from build123d import *

# Parameters (mm, degrees)
F0_W     = 50
F0_H     = 20
F1_DEPTH = 3


with BuildPart() as f1:
    # F0 (on Top) → F1 (new body)
    with BuildSketch(Plane.XY):
        Rectangle(F0_W, F0_H)
        Polygon((-13.6844948676, 3.9411129119), (-13.6844948676, -6.2236628849), (-16.3019989195, -6.2236628849), (-16.3019989195, 3.9411129119), (-19.6542409508, 3.9411129119), (-19.6542409508, 6.1183144246), (-10.3349540789, 6.1183144246), (-10.3349540789, 3.9411129119), align=None, mode=Mode.SUBTRACT)
        Polygon((-1.3290113452, -4.0626688277), (-1.3290113452, -6.2236628849), (-8.4359805511, -6.2236628849), (-8.4359805511, 6.1183144246), (-1.3290113452, 6.1183144246), (-1.3290113452, 3.9735278228), (-5.8184764992, 3.9735278228), (-5.8184764992, 1.2641815235), (-1.639654241, 1.2641815235), (-1.639654241, -0.8806050783), (-5.8184764992, -0.8806050783), (-5.8184764992, -4.0626688277), align=None, mode=Mode.SUBTRACT)
        with BuildLine():
            add(Edge.make_bspline(
                [(7.8889789303, -0.7576985413), (8.5305240411, -1.5883306321), (8.5305240411, -2.7957860616)],
                knots=[0, 0, 0, 1, 1, 1], degree=2))
            add(Edge.make_bspline(
                [(8.5305240411, -2.7957860616), (8.5305240411, -4.4678552134), (7.3271204754, -5.4308481902)],
                knots=[0, 0, 0, 1, 1, 1], degree=2))
            add(Edge.make_bspline(
                [(7.3271204754, -5.4308481902), (6.1237169098, -6.3938411669), (3.9816315505, -6.3938411669)],
                knots=[0, 0, 0, 1, 1, 1], degree=2))
            add(Edge.make_bspline(
                [(3.9816315505, -6.3938411669), (2.0043219881, -6.3938411669), (0.4862236629, -5.6482982172)],
                knots=[0, 0, 0, 1, 1, 1], degree=2))
            Line((0.4862236629, -5.6482982172), (0.4862236629, -3.2171799028))
            add(Edge.make_bspline(
                [(0.4862236629, -3.2171799028), (1.734197731, -3.7763371151), (2.5999459751, -4.0032414911)],
                knots=[0, 0, 0, 1, 1, 1], degree=2))
            add(Edge.make_bspline(
                [(2.5999459751, -4.0032414911), (3.4656942193, -4.2301458671), (4.1842247434, -4.2301458671)],
                knots=[0, 0, 0, 1, 1, 1], degree=2))
            add(Edge.make_bspline(
                [(4.1842247434, -4.2301458671), (5.0432198811, -4.2301458671), (5.5037817396, -3.9019448947)],
                knots=[0, 0, 0, 1, 1, 1], degree=2))
            add(Edge.make_bspline(
                [(5.5037817396, -3.9019448947), (5.9643435981, -3.5737439222), (5.9643435981, -2.9227444625)],
                knots=[0, 0, 0, 1, 1, 1], degree=2))
            add(Edge.make_bspline(
                [(5.9643435981, -2.9227444625), (5.9643435981, -2.5607779579), (5.7617504052, -2.2771474878)],
                knots=[0, 0, 0, 1, 1, 1], degree=2))
            add(Edge.make_bspline(
                [(5.7617504052, -2.2771474878), (5.5591572123, -1.9935170178), (5.1661264182, -1.7328471097)],
                knots=[0, 0, 0, 1, 1, 1], degree=2))
            add(Edge.make_bspline(
                [(5.1661264182, -1.7328471097), (4.773095624, -1.4721772015), (3.5656401945, -0.8968125338)],
                knots=[0, 0, 0, 1, 1, 1], degree=2))
            add(Edge.make_bspline(
                [(3.5656401945, -0.8968125338), (2.4365207996, -0.3646677472), (1.8706104808, 0.1242571583)],
                knots=[0, 0, 0, 1, 1, 1], degree=2))
            add(Edge.make_bspline(
                [(1.8706104808, 0.1242571583), (1.3047001621, 0.6131820637), (0.9670448406, 1.2641815235)],
                knots=[0, 0, 0, 1, 1, 1], degree=2))
            add(Edge.make_bspline(
                [(0.9670448406, 1.2641815235), (0.6293895192, 1.9151809833), (0.6293895192, 2.7822798487)],
                knots=[0, 0, 0, 1, 1, 1], degree=2))
            add(Edge.make_bspline(
                [(0.6293895192, 2.7822798487), (0.6293895192, 4.4219340897), (1.7396002161, 5.3579146407)],
                knots=[0, 0, 0, 1, 1, 1], degree=2))
            add(Edge.make_bspline(
                [(1.7396002161, 5.3579146407), (2.849810913, 6.2938951918), (4.8082117774, 6.2938951918)],
                knots=[0, 0, 0, 1, 1, 1], degree=2))
            add(Edge.make_bspline(
                [(4.8082117774, 6.2938951918), (5.7698541329, 6.2938951918), (6.6437061048, 6.0669908158)],
                knots=[0, 0, 0, 1, 1, 1], degree=2))
            add(Edge.make_bspline(
                [(6.6437061048, 6.0669908158), (7.5175580767, 5.8400864398), (8.4710967045, 5.4267963263)],
                knots=[0, 0, 0, 1, 1, 1], degree=2))
            Line((8.4710967045, 5.4267963263), (7.6283090222, 3.3900594273))
            add(Edge.make_bspline(
                [(7.6283090222, 3.3900594273), (6.639654241, 3.7952458131), (5.9940572663, 3.9559697461)],
                knots=[0, 0, 0, 1, 1, 1], degree=2))
            add(Edge.make_bspline(
                [(5.9940572663, 3.9559697461), (5.3484602917, 4.1166936791), (4.7244732577, 4.1166936791)],
                knots=[0, 0, 0, 1, 1, 1], degree=2))
            add(Edge.make_bspline(
                [(4.7244732577, 4.1166936791), (3.9816315505, 4.1166936791), (3.5845488925, 3.7709346299)],
                knots=[0, 0, 0, 1, 1, 1], degree=2))
            add(Edge.make_bspline(
                [(3.5845488925, 3.7709346299), (3.1874662345, 3.4251755808), (3.1874662345, 2.868719611)],
                knots=[0, 0, 0, 1, 1, 1], degree=2))
            add(Edge.make_bspline(
                [(3.1874662345, 2.868719611), (3.1874662345, 2.5229605619), (3.3481901675, 2.2649918963)],
                knots=[0, 0, 0, 1, 1, 1], degree=2))
            add(Edge.make_bspline(
                [(3.3481901675, 2.2649918963), (3.5089141005, 2.0070232307), (3.8587250135, 1.7666126418)],
                knots=[0, 0, 0, 1, 1, 1], degree=2))
            add(Edge.make_bspline(
                [(3.8587250135, 1.7666126418), (4.2085359265, 1.5262020529), (5.5159373312, 0.9022150189)],
                knots=[0, 0, 0, 1, 1, 1], degree=2))
            add(Edge.make_bspline(
                [(5.5159373312, 0.9022150189), (7.2474338196, 0.0729335494), (7.8889789303, -0.7576985413)],
                knots=[0, 0, 0, 1, 1, 1], degree=2))
        make_face(mode=Mode.SUBTRACT)
        Polygon((15.529443544, 3.9411129119), (15.529443544, -6.2236628849), (12.9119394922, -6.2236628849), (12.9119394922, 3.9411129119), (9.5596974608, 3.9411129119), (9.5596974608, 6.1183144246), (18.8789843328, 6.1183144246), (18.8789843328, 3.9411129119), align=None, mode=Mode.SUBTRACT)
    extrude(amount=F1_DEPTH)


solid = f1.part
The listing builds one solid part. Answer for the finished solid, in the listing's coordinates (mm). Round coordinates to 2 decimals unless told otherwise and drop trailing zeros. Order: outer loops, then holes, each group sorted by start corner. A loop starts at its lowest first (then second) coordinate and runs counter-clockwise, first axis right, second up. Notation, with made-up numbers: (81, -8) -> (102, -8) arc R33 ccw to (102, 23) -> close; hole circle Ø10 at (30, 61). An arc over 180 degrees is marked (long way). Put each result on its own line as item: value.
Q1. Consider line 1 along Y through (x, z) = (-11, 1.45); line 2 along Y through (x, z) = (1, 2); line 3 along X through (y, z) = (-2.5, 0.8). Determine where each line is inside the solid, lowest interval first.
Results list:
line 1: -10 to 3.94, 6.12 to 10
line 2: -10 to -5.87, -3.44 to 1.2, 4.44 to 10
line 3: -25 to -16.3, -13.68 to -8.44, -5.82 to 5.88, 8.52 to 12.91, 15.53 to 25
Q2. Determine the mould class of faces 1 (the flat face through (25, 0, 1)), 2 (the flat face through (0, -10, 1)), 3 (the flat face through (-1.64, 0, 1)) for opening direction Y: pulls with the +Y half, pulls with the -Y half, needs draft (parallel to the pull), parting line crosses it, or undercut.
Results list:
face 1: needs draft
face 2: pulls with the -Y half
face 3: undercut
Q3. Section C-C, the plane z = 0.95 is taken. Count the separate pieces of the cut face and the enclosed holes in it, and give its area (3 significant figures).
Results list:
separate pieces: 1
enclosed holes: 4
area: 788 mm^2
Q4. Section B-B, the plane x = -3 is taken. Write down the section's boundary in (y, z).
Results list:
outline: (-10, 0) -> (-6.22, 0) -> (-6.22, 3) -> (-10, 3) -> close; (-4.06, 0) -> (-0.88, 0) -> (-0.88, 3) -> (-4.06, 3) -> close; (1.26, 0) -> (3.97, 0) -> (3.97, 3) -> (1.26, 3) -> close; (6.12, 0) -> (10, 0) -> (10, 3) -> (6.12, 3) -> close
Q5. Section A-A, the plane x = 13.5 is taken. Write down the section's boundary in (y, z), and give its area (3 significant figures).
Results list:
outline: (-10, 0) -> (-6.22, 0) -> (-6.22, 3) -> (-10, 3) -> close; (6.12, 0) -> (10, 0) -> (10, 3) -> (6.12, 3) -> close
area: 23.0 mm^2
